Build history of the part. All positions in model axes, mm. A direction names the side the tool comes from. Coordinates: 2 decimals unless noted, no trailing zeros. Write each loop counter-clockwise with the first axis right and the second up, starting at its lowest first coordinate (ties: lowest second). Pieces come first, ordered by that corner, then holes. Notation, with made-up numbers: M -22.75,69.5 L -2.75,69.5 A28 ccw -2.75,102.5 Z; hole C 72.5,-11.5 d1. An arc over 180 degrees is marked long. Use CSV: the item, a comma, the result in double quotes. Start each with the question number.
```python
from build123d import *

# Parameters (mm, degrees)
SKETCH2_W           = 160
SKETCH2_H           = 110
BOSS_EXTRUDE1_DEPTH = 1.5
FILLET1_R           = 5
CUT_EXTRUDE1_DEPTH  = 4
FILLET2_R           = 2
FILLET3_R           = 4
CUT_EXTRUDE2_DEPTH  = 1.07
FILLET4_R           = 2


with BuildPart() as part:
    # Sketch2 → Boss-Extrude1 (new body, symmetric)
    with BuildSketch(Plane(origin=(0, 0, 0), x_dir=(1, 0, 0), z_dir=(0, 1, 0))):
        Rectangle(SKETCH2_W, SKETCH2_H)
    extrude(amount=BOSS_EXTRUDE1_DEPTH, both=True)

    # Fillet1
    fillet1_edges = [part.edges().sort_by_distance(p)[0] for p in [
        (80, 0, 55),
        (-80, 0, 55),
        (-80, 0, -55),
        (80, 0, -55),
    ]]
    fillet(fillet1_edges, radius=FILLET1_R)

    # Sketch3 → Cut-Extrude1 (cut, through all)
    with BuildSketch(Plane(origin=(0, 1.5, 0), x_dir=(1, 0, 0), z_dir=(0, 1, 0))):
        Polygon((-71, 2.5), (-51, 2.5), (-41, 2.5), (-41, 14.1), (23, 14.1), (23, -38.5), (-41, -38.5), (-41, -17), (-49.93, -17), (-51, -17), (-51, -20.5), (-71, -20.5), align=None)
    extrude(amount=-CUT_EXTRUDE1_DEPTH, mode=Mode.SUBTRACT)

    # Fillet2
    fillet2_edges = [part.edges().sort_by_distance(p)[0] for p in [
        (-51, 0, 20.5),
        (-71, 0, 20.5),
        (-71, 0, -2.5),
        (-41, 0, -2.5),
        (-41, 0, 17),
    ]]
    fillet(fillet2_edges, radius=FILLET2_R)

    # Fillet3
    fillet3_edges = [part.edges().sort_by_distance(p)[0] for p in [
        (-41, 0, -14.1),
        (23, 0, -14.1),
        (23, 0, 38.5),
        (-41, 0, 38.5),
    ]]
    fillet(fillet3_edges, radius=FILLET3_R)

    # Sketch4 → Cut-Extrude2 (cut)
    with BuildSketch(Plane(origin=(0, 1.5, 0), x_dir=(1, 0, 0), z_dir=(0, 1, 0))):
        with BuildLine():
            Line((-65.2, 2.5), (-65.2, 45))
            Line((-65.2, 45), (23, 45))
            Line((23, 45), (23, 10.1))
            ThreePointArc((23, 10.1), (21.828427125, 12.928427125), (19, 14.1))
            Line((19, 14.1), (-37, 14.1))
            ThreePointArc((-37, 14.1), (-39.828427125, 12.928427125), (-41, 10.1))
            Line((-41, 10.1), (-41, 9.5))
            Line((-41, 9.5), (30.1, 9.5))
            Line((30.1, 9.5), (30.1, -20.5))
            Line((30.1, -20.5), (-49.5, -20.5))
            Line((-49.5, -20.5), (-49.5, 2.5))
            Line((-49.5, 2.5), (-65.2, 2.5))
        make_face()
    extrude(amount=-CUT_EXTRUDE2_DEPTH, mode=Mode.SUBTRACT)

    # Fillet4
    fillet4_edges = [part.edges().sort_by_distance(p)[0] for p in [
        (-49.5, 0.965, 20.5),
        (-65.2, 0.965, -45),
        (23, 0.965, -45),
    ]]
    fillet(fillet4_edges, radius=FILLET4_R)


solid = part.part
```
1. 3-axis set-ups, long thin cutter, end or side, ignore diameter. For faces 1 (the flat face through (-9, 0, 38.5)), 2 (the flat face through (27, 0.43, 5)), 3 (the cylindrical face through (79, 0, 53)): which of +Z, -Z, +X, -X, +Y, -Y reach the whole face in a straight line?
2. Pull direction X, two halves, no side cores. Call faces 4 (the flat face through (-80, 0, 1)), 5 (the flat face through (34, 1.5, -1)), 6 (the flat face through (-71, 0, 9)): pulls with the +X half, pulls with the -X half, needs draft (parallel to the pull), parting line crosses it, or undercut.
3. Slice it at C-C (y = -0.1). List the corners of the cut face in (x, z), and give its area (3 significant figures).
4. Slice it at D-D (x = 26). List the corners of the cut face in (y, z), and give its area (3 significant figures).
5. Drill centre lines: line 1 along X through (y, z) = (-1.05, 11.5); line 2 along X through (y, z) = (-0.65, 20); line 3 along Z through (x, y) = (-54.5, 0.2). Where is each one in solid material? Low to high. Write a range as from..to.
6. Flat gauge pin, fed straight in: pin 1 (13 mm diameter, centred on x = -5, z = -29, fed in from +Y). Where does the tip first touch, or does it go through?
7. Slice it at B-B (x = -21.5). List the corners of the cut face in (y, z), and give its area (3 significant figures).
8. Slice it at A-A (z = 27). List the corners of the cut face in (x, y).
Established:
1,face 1,"+Y, -Y"
1,face 2,"+Y"
1,face 3,"+Z, +X, +Y, -Y"
2,face 4,"pulls with the -X half"
2,face 5,"needs draft"
2,face 6,"undercut"
3,outline,"M -80,-50 A5 ccw -75,-55 L 75,-55 A5 ccw 80,-50 L 80,50 A5 ccw 75,55 L -75,55 A5 ccw -80,50 Z; hole M -71,-0.5 A2 ccw -69,-2.5 L -43,-2.5 A2 cw -41,-4.5 L -41,-10.1 A4 ccw -37,-14.1 L 19,-14.1 A4 ccw 23,-10.1 L 23,34.5 A4 ccw 19,38.5 L -37,38.5 A4 ccw -41,34.5 L -41,19 A2 cw -43,17 L -51,17 L -51,18.5 A2 ccw -53,20.5 L -69,20.5 A2 ccw -71,18.5 Z"
3,area,"13,600 mm2"
4,outline,"M -1.5,-55 L 1.5,-55 L 1.5,-9.5 L 0.43,-9.5 L 0.43,20.5 L 1.5,20.5 L 1.5,55 L -1.5,55 Z"
4,area,"298 mm2"
5,line 1,"x = -80..-71, 23..80"
5,line 2,"x = -80..-70.32, -51.68..-41, 23..80"
5,line 3,"z = -55..-2.5, 20.5..55"
6,pin 1,"stops at y = 0.43"
7,outline,"M -1.5,-55 L 1.5,-55 L 1.5,-45 L 0.43,-45 L 0.43,-14.1 L -1.5,-14.1 Z; M -1.5,38.5 L 1.5,38.5 L 1.5,55 L -1.5,55 Z"
7,area,"139 mm2"
8,outline,"M -80,-1.5 L -41,-1.5 L -41,1.5 L -80,1.5 Z; M 23,-1.5 L 80,-1.5 L 80,1.5 L 23,1.5 Z"
